The model under review builds one solid part; all positions refer to its coordinate system, in mm. A direction names the side the tool comes from. Coordinates: 2 decimals unless noted, no trailing zeros. Loops run counter-clockwise (first coordinate to the right, second up) from the corner with the lowest first, then second, coordinate; pieces in that order, holes last. Notation, with made-up numbers: (-38, 73) - (-13, 73) arc R34 ccw to (-13, 111) - close; hole circle Ø8 at (11, 52). An arc over 180 degrees is marked (long way). Answer in a Markdown table with one row per item. Add a question column.
(1) We need section C-C on x = -35. Write out the cut boundary in (y, z), plus the area to 3 significant figures.
(2) For P1, Ø5, axis at y = 28.5, z = 6, coming from the +X side; P2, Ø14.5, axis at x = -44.5, y = -27.5, coming from the -Z side; P3, Ø6.5, axis at x = -43.5, y = 29, coming from the -Z side; P4, Ø3, axis at x = -16.5, z = 12.5, coming from the -Y side, all flat-tipped, find the tip position at first contact; note any pin that passes through.
(3) Mouldability with a two-part tool opening along Y and no side actions: class faces 1 (the cylindrical face through (-17.58, -32.53, 22.62)), 2 (the cylindrical face through (-8.07, 26.5, 0.07)), 3 (the cylindrical face through (-36.43, -36.13, 8.55)), 4 (the cylindrical face through (-43.503, 0.286, 4.86)) as +Y half, -Y half, draft (parallel to the pull), parting line (faces both ways), or undercut.
(4) Machinability: for faces 5 (the cylindrical face through (22.58, 19.15, -2.54)), 6 (the flat face through (-31.5, -45.3, 2.6)), 7 (the flat face through (-31.5, 0, 33)), 8 (the cylindrical face through (-1.773, -12.918, 2.465)), which of the approach directions +Z, -Z, +X, -X, +Y, -Y give a long, thin tool a straight path to every point of the face, cutting with its end or side? Answer none if there is none.
(5) For line 1 along X through (y, z) = (-15, -1.85); line 2 along X through (y, z) = (-15, 3.8); line 3 along Y through (x, z) = (-36.5, 8), list the stretches that pass through material, from the lowest coordinate up.
(6) We need section B-B on x = -1.5. Write out the cut boundary in (y, z), plus the area to 3 significant figures.
(7) We need section A-A on y = 15. Write out the cut boundary in (x, z).
(8) We need section D-D on y = 0. Write out the cut boundary in (x, z).
from build123d import *

# Parameters (mm, degrees)
SKETCH_R        = 2.1
PAD_DEPTH       = 5
SKETCH001_W     = 10
SKETCH001_H     = 50
PAD001_DEPTH    = 30
SKETCH002_W     = 22
SKETCH002_H     = 40
SKETCH002_R     = 2.6
PAD002_DEPTH    = 10
SKETCH004_R     = 5
POCKET001_DEPTH = 5
FILLET_R        = 5
SKETCH003_R     = 4.25
POCKET_DEPTH    = 5
PAD003_DEPTH    = 20
SKETCH006_R     = 2.75
POCKET002_DEPTH = 359.065568
SKETCH007_R     = 5.25
POCKET003_DEPTH = 10
CHAMFER_SIZE2   = 16
CHAMFER_SIZE    = 10
FILLET001_R     = 9
SKETCH008_R     = 6.5
POCKET004_DEPTH = 4


with BuildPart() as part:
    # Sketch → Pad (new body, symmetric)
    with BuildSketch(Plane.XY):
        with BuildLine():
            Line((-31.5, -25), (-31.5, 25))
            Line((-31.5, 25), (3.702041, 25))
            ThreePointArc((3.702041, 25), (13.5, 17), (23.297959, 25))
            Line((31.5, 25), (23.297959, 25))
            Line((31.5, 25), (31.5, -25))
            Line((23.297959, -25), (31.5, -25))
            ThreePointArc((23.297959, -25), (13.5, -17), (3.702041, -25))
            Line((-31.5, -25), (3.702041, -25))
        make_face()
        with Locations((-1.5, 15)):
            Circle(SKETCH_R, mode=Mode.SUBTRACT)
        with Locations((23.5, 15)):
            Circle(SKETCH_R, mode=Mode.SUBTRACT)
        with Locations((23.5, -15)):
            Circle(SKETCH_R, mode=Mode.SUBTRACT)
        with Locations((-1.5, -15)):
            Circle(SKETCH_R, mode=Mode.SUBTRACT)
    extrude(amount=PAD_DEPTH, both=True)

    # Sketch001 (on Face14 of Pad) → Pad001 (join)
    with BuildSketch(Plane.XY.offset(5)):
        with Locations((-26.5, 0)):
            Rectangle(SKETCH001_W, SKETCH001_H)
    extrude(amount=PAD001_DEPTH)

    # Sketch002 (on Face8 of Pad001) → Pad002 (join)
    with BuildSketch(Plane.XZ.offset(25)):
        with Locations((-20.5, 15)):
            Rectangle(SKETCH002_W, SKETCH002_H)
        with Locations((-16.5, 27.5)):
            Circle(SKETCH002_R, mode=Mode.SUBTRACT)
        with Locations((-16.5, 12.5)):
            Circle(SKETCH002_R, mode=Mode.SUBTRACT)
    pad002 = extrude(amount=PAD002_DEPTH)

    # Sketch004 (on Face20 of Pad002) → Pocket001 (cut)
    with BuildSketch(Plane.XZ.offset(35)):
        with Locations((-16.5, 27.5)):
            Circle(SKETCH004_R)
        with Locations((-16.5, 12.5)):
            Circle(SKETCH004_R)
    pocket001 = extrude(amount=-POCKET001_DEPTH, mode=Mode.SUBTRACT)

    # Mirrored: Pad002, Pocket001 across XZ
    add(pad002.mirror(Plane.XZ))
    add(pocket001.mirror(Plane.XZ), mode=Mode.SUBTRACT)

    # Fillet
    fillet_edges = [part.edges().sort_by_distance(p)[0] for p in [
        (-9.5, 25, 0),
        (-9.5, -25, 0),
    ]]
    fillet(fillet_edges, radius=FILLET_R)

    # Sketch003 (on Face2 of Fillet) → Pocket (cut)
    with BuildSketch(Plane(origin=(0, 0, -5), x_dir=(1, 0, 0), z_dir=(0, 0, -1))):
        with Locations((-1.5, 15)):
            Circle(SKETCH003_R)
        with Locations((23.5, 15)):
            Circle(SKETCH003_R)
        with Locations((23.5, -15)):
            Circle(SKETCH003_R)
        with Locations((-1.5, -15)):
            Circle(SKETCH003_R)
    extrude(amount=-POCKET_DEPTH, mode=Mode.SUBTRACT)

    # Sketch005 (on Face2 of Pocket) → Pad003 (join)
    with BuildSketch(Plane(origin=(0, 0, -5), x_dir=(1, 0, 0), z_dir=(0, 0, -1))):
        with BuildLine():
            ThreePointArc((-56.5, -13), (-43.5, 0), (-56.5, 13))
            Line((-56.5, 13), (-56.5, 47.5))
            Line((-56.5, 47.5), (-31.5, 47.5))
            Line((-31.5, -47.5), (-31.5, 47.5))
            Line((-56.5, -47.5), (-31.5, -47.5))
            Line((-56.5, -13), (-56.5, -47.5))
        make_face()
    extrude(amount=-PAD003_DEPTH)

    # Sketch006 (on Face35 of Pad003) → Pocket002 (cut, through all)
    with BuildSketch(Plane(origin=(-56.5, 0, 0), x_dir=(0, -1, 0), z_dir=(-1, 0, 0))):
        with Locations((-40, 5)):
            Circle(SKETCH006_R)
    pocket002 = extrude(amount=-POCKET002_DEPTH, mode=Mode.SUBTRACT)

    # Sketch007 (on Face32 of Pocket002) → Pocket003 (cut)
    with BuildSketch(Plane.YZ.offset(-31.5)):
        with Locations((40, 5)):
            Circle(SKETCH007_R)
    pocket003 = extrude(amount=-POCKET003_DEPTH, mode=Mode.SUBTRACT)

    # Mirrored001: Pocket002, Pocket003 across Sketch006 V_Axis
    add(pocket002.mirror(Plane(origin=(-56.5, 0, 0), x_dir=(-1, 0, 0), z_dir=(0, -1, 0))), mode=Mode.SUBTRACT)
    add(pocket003.mirror(Plane(origin=(-56.5, 0, 0), x_dir=(-1, 0, 0), z_dir=(0, -1, 0))), mode=Mode.SUBTRACT)

    # Chamfer
    chamfer_edges = [part.edges().sort_by_distance(p)[0] for p in [
        (-31.5, 0, 15),
    ]]
    chamfer_side = part.faces().sort_by_distance((-43.121304, 0, 15))[0]
    chamfer(chamfer_edges, length=CHAMFER_SIZE, length2=CHAMFER_SIZE2, reference=chamfer_side)

    # Fillet001
    fillet001_edges = [part.edges().sort_by_distance(p)[0] for p in [
        (-44, 47.5, 15),
        (-44, 47.5, -5),
        (-44, -47.5, 15),
        (-44, -47.5, -5),
    ]]
    fillet(fillet001_edges, radius=FILLET001_R)

    # Sketch008 (on Face14 of Fillet001) → Pocket004 (cut)
    with BuildSketch(Plane(origin=(0, 0, -5), x_dir=(1, 0, 0), z_dir=(0, 0, -1))):
        with Locations((-44, 30)):
            Circle(SKETCH008_R)
        with Locations((16, 0)):
            Circle(SKETCH008_R)
        with Locations((-44, -30)):
            Circle(SKETCH008_R)
    extrude(amount=-POCKET004_DEPTH, mode=Mode.SUBTRACT)


solid = part.part
Outcome:
| question | item | result |
|---|---|---|
| 1 | outline | (-47.5, 4) arc R9 ccw to (-38.5, -5) - (38.5, -5) arc R9 ccw to (47.5, 4) - (47.5, 6) arc R9 ccw to (38.5, 15) - (35, 15) - (35, 25.4) - (-35, 25.4) - (-35, 15) - (-38.5, 15) arc R9 ccw to (-47.5, 6) - close; hole circle Ø10.5 at (-40, 5); hole circle Ø10.5 at (40, 5) |
| 1 | area | 2,390 mm² |
| 2 | P1 | x = -7.76 |
| 2 | P2 | z = -5 |
| 2 | P3 | z = -1 |
| 2 | P4 | through |
| 3 | face 1 | draft |
| 3 | face 2 | +Y half |
| 3 | face 3 | undercut |
| 3 | face 4 | undercut |
| 4 | face 5 | -Z |
| 4 | face 6 | +Z, -Z, +X, -Y |
| 4 | face 7 | +Z, -X, +Y, -Y |
| 4 | face 8 | +Z, -Z |
| 5 | line 1 | -56.5 to -5.75, 2.75 to 19.25, 27.75 to 31.5 |
| 5 | line 2 | -56.5 to -3.6, 0.6 to 21.4, 25.6 to 31.5 |
| 5 | line 3 | -47.27 to -44.31, -35.69 to 35.69, 44.31 to 47.27 |
| 6 | outline | (-25, -5) - (-19.25, -5) - (-19.25, 0) - (-17.1, 0) - (-17.1, 5) - (-25, 5) - close; (-12.9, 0) - (-10.75, 0) - (-10.75, -5) - (10.75, -5) - (10.75, 0) - (12.9, 0) - (12.9, 5) - (-12.9, 5) - close; (17.1, 0) - (19.25, 0) - (19.25, -5) - (25, -5) - (25, 5) - (17.1, 5) - close |
| 6 | area | 373 mm² |
| 7 | outline | (-56.5, -5) - (-5.75, -5) - (-5.75, 0) - (-3.6, 0) - (-3.6, 5) - (-21.5, 5) - (-21.5, 35) - (-31.5, 35) - (-31.5, 31) - (-41.5, 15) - (-56.5, 15) - close; (0.6, 0) - (2.75, 0) - (2.75, -5) - (19.25, -5) - (19.25, 0) - (21.4, 0) - (21.4, 5) - (0.6, 5) - close; (25.6, 0) - (27.75, 0) - (27.75, -5) - (31.5, -5) - (31.5, 5) - (25.6, 5) - close |
| 8 | outline | (-43.5, -5) - (9.5, -5) - (9.5, -1) - (22.5, -1) - (22.5, -5) - (31.5, -5) - (31.5, 5) - (-21.5, 5) - (-21.5, 35) - (-31.5, 35) - (-31.5, 31) - (-41.5, 15) - (-43.5, 15) - close |
